Part model, mm, in its own coordinate system. A direction names the side the tool comes from. Round coordinates to 2 decimals unless told otherwise and drop trailing zeros. Write each loop counter-clockwise with the first axis right and the second up, starting at its lowest first coordinate (ties: lowest second). Pieces come first, ordered by that corner, then holes. Notation, with made-up numbers: M 42.25,11.25 L 71.25,11.25 A14 ccw 71.25,23.25 Z; hole C -27.75,57.25 d1. An arc over 180 degrees is marked long. Use a Markdown table: item, result. Add a question column.
1) Slice it at C-C on y = -3.5. Write the cut outline in (x, z).
2) Drop flat-ended pins along their axis: P1, Ø1, axis at x = -1, y = -11.5, coming from the -Z side; P2, Ø0.9, axis at y = 16, z = 8, coming from the +X side; P3, Ø6, axis at y = 7.5, z = 7.5, coming from the +X side. Give the stop position or say it passes through.
3) Slice it at B-B on z = 8.75. Write the cut outline in (x, y), plus the area to 3 significant figures.
4) Slice it at D-D on x = 12.5. Write the cut outline in (y, z), plus the area to 3 significant figures.
5) Slice it at A-A on x = 0. Write the cut outline in (y, z), plus the area to 3 significant figures.
6) Wall check: probe 1 along Y at (x, z) = (0, 0.95); probe 2 along Y at (x, z) = (0, 7.5); probe 3 along Z at (x, y) = (-13.5, -10). Give the ranges that are in metal, low to high.
7) Which spindle directions (+Z, -Z, +X, -X, +Y, -Y) get a long thin tool onto all of the face, cutting with end or side? Do faces 5 (the face through (-0.228, 9.265, 1.528)), 6 (the face through (-0.16, 9.76, 8.97)), 7 (the face through (1.5, 16, 5)). Say none if no direction does.
8) Two-plate mould, pull along X, no slides. Class faces 1 (the face through (0, 17.95, 7)), 2 (the face through (-1.5, 16, 5)), 3 (the face through (-0.636, -14.936, 5.423)), 4 (the face through (1, -10, 3.1)): released by +X, released by -X, zero draft, split by the parting line, or undercut.
```python
from build123d import *

# Parameters (mm, degrees)
F1_DEPTH = 11
F3_DEPTH = 4
F4_R     = 7.5
F5_DEPTH = 25
F6_R     = 1.25
F7_DEPTH = 25
F6_R_2   = 1.75
F8_DEPTH = 3.1


with BuildPart() as f1:
    # F0 (on Top) → F1 (new body)
    with BuildSketch(Plane.XY):
        with BuildLine():
            Line((-1.5, 17.95), (-1.5, 14.874559))
            ThreePointArc((-1.5, 14.874559), (0, -14.95), (1.5, 14.874559))
            Line((1.5, 14.874559), (1.5, 17.95))
            Line((1.5, 17.95), (-1.5, 17.95))
        make_face()
    extrude(amount=F1_DEPTH)

    # F2 (on face) → F3 (join)
    with BuildSketch(Plane.XY.offset(11)):
        with BuildLine():
            ThreePointArc((-1.5, 17.95), (-12.194951, -13.256533), (18.012565, 0))
            ThreePointArc((18.012565, 0), (13.256533, 12.194951), (1.5, 17.95))
            Line((1.5, 17.95), (1.5, 14.874559))
            ThreePointArc((1.5, 14.874559), (0, -14.95), (-1.5, 14.874559))
            Line((-1.5, 14.874559), (-1.5, 17.95))
        make_face()
        with BuildLine():
            Line((1.5, 14.874559), (1.5, 17.95))
            Line((1.5, 17.95), (-1.5, 17.95))
            Line((-1.5, 17.95), (-1.5, 14.874559))
            ThreePointArc((-1.5, 14.874559), (0, -14.95), (1.5, 14.874559))
        make_face()
    extrude(amount=F3_DEPTH)

    # F4 (on face) → F5 (cut)
    with BuildSketch(Plane(origin=(0, 0, 0), x_dir=(1, 0, 0), z_dir=(0, 0, -1))):
        Circle(F4_R)
    extrude(amount=-F5_DEPTH, mode=Mode.SUBTRACT)

    # F6 (on face) → F7 (cut)
    with BuildSketch(Plane(origin=(0, 0, 0), x_dir=(1, 0, 0), z_dir=(0, 0, -1))):
        with Locations((0, -11)):
            Circle(F6_R)
        with Locations((0, 11)):
            Circle(F6_R)
    extrude(amount=-F7_DEPTH, mode=Mode.SUBTRACT)

    # F6 (on face) → F8 (cut)
    with BuildSketch(Plane(origin=(0, 0, 0), x_dir=(1, 0, 0), z_dir=(0, 0, -1))):
        with Locations((0, 11)):
            Circle(F6_R_2)
        with Locations((0, 11)):
            Circle(F6_R, mode=Mode.SUBTRACT)
        with Locations((0, -11)):
            Circle(F6_R_2)
        with Locations((0, -11)):
            Circle(F6_R, mode=Mode.SUBTRACT)
    extrude(amount=-F8_DEPTH, mode=Mode.SUBTRACT)


solid = f1.part
```
Entries:
| question | item | result |
|---|---|---|
| 1 | outline | M -17.67,11 L -14.53,11 L -14.53,0 L -6.63,0 L -6.63,15 L -17.67,15 Z; M 6.63,0 L 14.53,0 L 14.53,11 L 17.67,11 L 17.67,15 L 6.63,15 Z |
| 2 | P1 | stops at z = 3.1 |
| 2 | P2 | stops at x = 1.5 |
| 2 | P3 | stops at x = 14.26 |
| 3 | outline | M -1.5,14.87 A14.95 ccw long 1.5,14.87 L 1.5,17.95 L -1.5,17.95 Z; hole C 0,0 d15; hole C 0,-11 d2.5; hole C 0,11 d2.5 |
| 3 | area | 525 mm^2 |
| 4 | outline | M -12.97,11 L -8.2,11 L -8.2,0 L 8.2,0 L 8.2,11 L 12.97,11 L 12.97,15 L -12.97,15 Z |
| 4 | area | 284 mm^2 |
| 5 | outline | M -18.01,11 L -14.95,11 L -14.95,0 L -12.75,0 L -12.75,3.1 L -12.25,3.1 L -12.25,15 L -18.01,15 Z; M -9.75,3.1 L -9.25,3.1 L -9.25,0 L -7.5,0 L -7.5,15 L -9.75,15 Z; M 7.5,0 L 9.25,0 L 9.25,3.1 L 9.75,3.1 L 9.75,15 L 7.5,15 Z; M 12.25,3.1 L 12.75,3.1 L 12.75,0 L 17.95,0 L 17.95,15 L 12.25,15 Z |
| 5 | area | 200 mm^2 |
| 6 | probe 1 | y = -14.95 to -12.75, -9.25 to -7.5, 7.5 to 9.25, 12.75 to 17.95 |
| 6 | probe 2 | y = -14.95 to -12.25, -9.75 to -7.5, 7.5 to 9.75, 12.25 to 17.95 |
| 6 | probe 3 | z = 11 to 15 |
| 7 | face 5 | -Z |
| 7 | face 6 | +Z, -Z |
| 7 | face 7 | -Z, +X, +Y |
| 8 | face 1 | zero draft |
| 8 | face 2 | released by -X |
| 8 | face 3 | split by the parting line |
| 8 | face 4 | undercut |
